```python
from build123d import *

# Parameters (mm, degrees)
F0_R     = 8
F1_DEPTH = 4
F2_R     = 7
F3_DEPTH = 12
F4_R     = 1.5
F5_DEPTH = 16.001
F6_R     = 0.025
F7_DEPTH = 5


with BuildPart() as f1:
    # F0 (on Front) → F1 (new body)
    with BuildSketch(Plane.XZ):
        Circle(F0_R)
    extrude(amount=F1_DEPTH)

    # F2 (on face) → F3 (join)
    with BuildSketch(Plane.XZ.offset(4)):
        Circle(F2_R)
    extrude(amount=F3_DEPTH)

    # F4 (on face) → F5 (cut, through all)
    with BuildSketch(Plane(origin=(0, 0, 0), x_dir=(-1, 0, 0), z_dir=(0, 1, 0))):
        Circle(F4_R)
    extrude(amount=-F5_DEPTH, mode=Mode.SUBTRACT)

    # F6 (on face) → F7 (cut)
    with BuildSketch(Plane(origin=(0, 0, 0), x_dir=(-1, 0, 0), z_dir=(0, 1, 0))):
        with Locations((-3.991511, 0.260457)):
            Circle(F6_R)
    extrude(amount=-F7_DEPTH, mode=Mode.SUBTRACT)


solid = f1.part
```
Can you work these out from the model? Positions are in its coordinate system, mm. A direction names the side the tool comes from. Coordinates: 2 decimals unless noted, no trailing zeros. Loops run counter-clockwise (first coordinate to the right, second up) from the corner with the lowest first, then second, coordinate; pieces in that order, holes last. Notation, with made-up numbers: M 7.25,6.25 L 29.25,6.25 A18 ccw 29.25,11.25 Z; hole C -20,47 d7. An arc over 180 degrees is marked long. Put each result on its own line as item: value. Start each with the question number.
(1) Imagine slicing it at C-C on y = -10. List the corners of the cut face in (x, z) for me, and give its area (3 significant figures).
(2) Which directions (+Z, -Z, +X, -X, +Y, -Y) give clear straight access to the entire face, cutting with the end or side of a thin tool? Please do faces 1 (the face through (2, 0, 0)), 2 (the face through (4, -4, -6)).
(3) Imagine slicing it at A-A on z = 0. List the corners of the cut face in (x, y) for me.
(4) I need wall thicknesses on probe 1 along X at (y, z) = (-4.75, -0.75); probe 2 along Y at (x, z) = (-6.5, -4.25); probe 3 along Z at (x, y) = (-2.5, -12.5). Which ranges of each line are inside material? Lowest first, please.
(5) Imagine slicing it at D-D on x = -5. List the corners of the cut face in (y, z) for me (3 decimals).
(6) Will these pins go through, and if not, where does the flat tip stop? pin 1 Ø4 at (x, y) = (-5.5, -9.5) entering from +Z; pin 2 Ø2 at (x, y) = (-4, -5.5) entering from -Z; pin 3 Ø1 at (x, y) = (-5.5, -3) entering from +Z (3 decimals).
(7) Imagine slicing it at B-B on x = 0. List the corners of the cut face in (y, z) for me.
(8) We'd pull the mould along Z, two halves only. Please class faces 3 (the face through (0, -16, 2)), 4 (the face through (-1.73, -1.97, -7.81)), 5 (the face through (1.5, -7.89, 0.07)): +Z half, -Z half, draft (parallel to the pull), parting line (faces both ways), or undercut.
Worked answers:
1. outline: C 0,0 d14; hole C 0,0 d3
1. area: 147 mm2
2. face 1: +Z, -Z, +X, -X, +Y
2. face 2: -Y
3. outline: M -8,-4 L -7,-4 L -7,-16 L -1.5,-16 L -1.5,0 L -8,0 Z; M 1.5,-16 L 7,-16 L 7,-4 L 8,-4 L 8,0 L 1.5,0 Z
4. probe 1: x = -6.96 to -1.3, 1.3 to 6.96
4. probe 2: y = -4 to 0
4. probe 3: z = -6.54 to 6.54
5. outline: M -16,-4.899 L -4,-4.899 L -4,-6.245 L 0,-6.245 L 0,6.245 L -4,6.245 L -4,4.899 L -16,4.899 Z
6. pin 1: stops at z = 6.06
6. pin 2: stops at z = -6.32
6. pin 3: stops at z = 6.245
7. outline: M -16,-7 L -4,-7 L -4,-8 L 0,-8 L 0,-1.5 L -16,-1.5 Z; M -16,1.5 L 0,1.5 L 0,8 L -4,8 L -4,7 L -16,7 Z
8. face 3: draft
8. face 4: parting line
8. face 5: undercut
